For this review, take the finished solid that the model builds, in its own axes (mm). Face numbers are marked on the shaded views. Coordinates: 2 decimals unless noted, no trailing zeros. Write each loop counter-clockwise with the first axis right and the second up, starting at its lowest first coordinate (ties: lowest second). Pieces come first, ordered by that corner, then holes. Notation, with made-up numbers: (58.25, -11.5) -> (73.25, -11.5) arc R26 ccw to (73.25, 26.5) -> close; hole circle Ø11 at (-34.5, -9.75). An arc over 180 degrees is marked (long way). Put each result on its own line as item: value. Start each with the question number.
Item 1: To check wall thickness, follow L1, parallel to Y at x = -19, z = 2.95; L2, parallel to Z at x = 49.5, y = 0.9; L3, parallel to X at y = -32, z = 2. State the ranges of each line that lie inside material, in increasing order.
Item 2: Consider section B-B on y = 12. Give the boundary of the cut face in (x, z), and give its area (3 significant figures).
Item 3: Consider section C-C on x = -37. Give the boundary of the cut face in (y, z).
Item 4: Consider section A-A on z = 2.75. Give the boundary of the cut face in (x, y).
Item 5: Insertion check: P1, Ø1.5, axis at x = 49, z = 4, coming from the -Y side; P2, Ø1.2, axis at y = -8, z = 3, coming from the +X side; P3, Ø1.5, axis at x = 49.5, z = 3.5, coming from the +Y side; P4, Ø4, axis at x = -1.5, y = 33.5, coming from the -Z side. Each pin has a flat end and moves straight along its axis. Give the tip position at first contact, or say it passes through.
Item 6: The part is to be moulded in two halves that separate along Y. For the marked faces 1 and 2, say which applies: +Y half, -Y half, draft (parallel to the pull), parting line (faces both ways), or undercut.
```python
from build123d import *

# Parameters (mm, degrees)
SKETCH1_W           = 88
SKETCH1_H           = 103
BOSS_EXTRUDE1_DEPTH = 5.5
SHELL1_T            = -1.25
SKETCH2_W           = 5
SKETCH2_H           = 10
BOSS_EXTRUDE2_DEPTH = 8
FILLET1_RADIUS      = 2.5
FILLET1_LENGTH      = 10
SKETCH3_R           = 1.5
CUT_EXTRUDE1_DEPTH  = 3
FILLET2_R           = 1.5


with BuildPart() as part:
    # Sketch1 → Boss-Extrude1 (new body)
    with BuildSketch(Plane.XY):
        Rectangle(SKETCH1_W, SKETCH1_H)
    extrude(amount=BOSS_EXTRUDE1_DEPTH)

    # Shell1
    shell1_openings = [part.faces().sort_by_distance(p)[0] for p in [
        (0, 0, 5.5),
    ]]
    offset(amount=SHELL1_T, openings=shell1_openings, kind=Kind.INTERSECTION)

    # Sketch2 → Boss-Extrude2 (add)
    with BuildSketch(Plane(origin=(44, 0, 0), x_dir=(0, 0, -1), z_dir=(1, 0, 0))):
        with Locations((-2.75, 5)):
            Rectangle(SKETCH2_W, SKETCH2_H)
    extrude(amount=BOSS_EXTRUDE2_DEPTH)

    # Fillet1: full round fillet: the end face becomes a half cylinder, R = half its width
    fillet1_face = Plane((52, 5, 2.75), x_dir=(0, 1, 0), z_dir=(1, 0, 0))  # on the end face: x along it, z out of the body
    fillet1_slab = fillet1_face.offset(-FILLET1_RADIUS / 2) * Box(FILLET1_LENGTH, 2 * FILLET1_RADIUS, FILLET1_RADIUS, mode=Mode.PRIVATE)  # the body's end, R deep
    fillet1_round = Plane((49.5, 5, 2.75), x_dir=(1, 0, 0), z_dir=(0, 1, 0)) * Cylinder(FILLET1_RADIUS, FILLET1_LENGTH, mode=Mode.PRIVATE)  # its axis R under the face
    add(fillet1_slab - fillet1_round, mode=Mode.SUBTRACT)

    # Sketch3 → Cut-Extrude1 (cut)
    with BuildSketch(Plane.XZ):
        with Locations((49.5, 2.75)):
            Circle(SKETCH3_R)
    extrude(amount=-CUT_EXTRUDE1_DEPTH, mode=Mode.SUBTRACT)

    # Fillet2
    # the kernel refuses this fillet: 1.5 mm, written as the material it takes off along each edge
    with BuildSketch(Plane(origin=(-42.5, -50, 1.5), x_dir=(0, 0, -1), z_dir=(-1, 0, 0))) as fillet2_piece_1_section:
        Polygon((0, 0), (FILLET2_R, 0), (FILLET2_R, FILLET2_R), (0, FILLET2_R), align=None)
    fillet2_piece_1 = extrude(amount=FILLET2_R, mode=Mode.PRIVATE)
    fillet2_piece_1 = fillet2_piece_1 - Plane(origin=(-42.5, -50, 1.5), x_dir=(0, 0.7071067811865475, 0.7071067811865475), z_dir=(-1, 0, 0)) * Sphere(FILLET2_R, mode=Mode.PRIVATE)
    add(fillet2_piece_1, mode=Mode.SUBTRACT)
    with BuildSketch(Plane(origin=(-42.5, 50, 1.5), x_dir=(-1, 0, 0), z_dir=(0, 1, 0))) as fillet2_piece_2_section:
        Polygon((0, 0), (FILLET2_R, 0), (FILLET2_R, -FILLET2_R), (0, -FILLET2_R), align=None)
    fillet2_piece_2 = extrude(amount=FILLET2_R, mode=Mode.PRIVATE)
    fillet2_piece_2 = fillet2_piece_2 - Plane(origin=(-42.5, 50, 1.5), x_dir=(0.7071067811865475, 0, 0.7071067811865475), z_dir=(0, 1, 0)) * Sphere(FILLET2_R, mode=Mode.PRIVATE)
    add(fillet2_piece_2, mode=Mode.SUBTRACT)
    with BuildSketch(Plane(origin=(42.5, -50, 1.5), x_dir=(0, 0, -1), z_dir=(1, 0, 0))) as fillet2_piece_3_section:
        Polygon((0, 0), (FILLET2_R, 0), (FILLET2_R, -FILLET2_R), (0, -FILLET2_R), align=None)
    fillet2_piece_3 = extrude(amount=FILLET2_R, mode=Mode.PRIVATE)
    fillet2_piece_3 = fillet2_piece_3 - Plane(origin=(42.5, -50, 1.5), x_dir=(0, 0.7071067811865475, 0.7071067811865475), z_dir=(1, 0, 0)) * Sphere(FILLET2_R, mode=Mode.PRIVATE)
    add(fillet2_piece_3, mode=Mode.SUBTRACT)
    with BuildSketch(Plane(origin=(42.5, 50, 1.5), x_dir=(1, 0, 0), z_dir=(0, 1, 0))) as fillet2_piece_4_section:
        Polygon((0, 0), (FILLET2_R, 0), (FILLET2_R, FILLET2_R), (0, FILLET2_R), align=None)
    fillet2_piece_4 = extrude(amount=FILLET2_R, mode=Mode.PRIVATE)
    fillet2_piece_4 = fillet2_piece_4 - Plane(origin=(42.5, 50, 1.5), x_dir=(-0.7071067811865475, 0, 0.7071067811865475), z_dir=(0, 1, 0)) * Sphere(FILLET2_R, mode=Mode.PRIVATE)
    add(fillet2_piece_4, mode=Mode.SUBTRACT)
    with BuildSketch(Plane(origin=(-44, -50, 0), x_dir=(0, 0, 1), z_dir=(0, 1, 0))) as fillet2_piece_5:
        with BuildLine():
            CenterArc((FILLET2_R, FILLET2_R), FILLET2_R, 180, 90)
            Line((0, FILLET2_R), (0, 0))
            Line((0, 0), (FILLET2_R, 0))
        make_face()
    extrude(amount=100, mode=Mode.SUBTRACT)
    with BuildSketch(Plane(origin=(42.5, -51.5, 0), x_dir=(0, 1, 0), z_dir=(-1, 0, 0))) as fillet2_piece_6:
        with BuildLine():
            CenterArc((FILLET2_R, -FILLET2_R), FILLET2_R, 90, 90)
            Line((0, -FILLET2_R), (0, 0))
            Line((0, 0), (FILLET2_R, 0))
        make_face()
    extrude(amount=85, mode=Mode.SUBTRACT)
    with BuildSketch(Plane(origin=(44, 50, 0), x_dir=(0, 0, 1), z_dir=(0, -1, 0))) as fillet2_piece_7_section:
        with BuildLine():
            CenterArc((FILLET2_R, FILLET2_R), FILLET2_R, 180, 90)
            Line((0, FILLET2_R), (0, 0))
            Line((0, 0), (FILLET2_R, 0))
        make_face()
    fillet2_piece_7 = extrude(amount=100, mode=Mode.PRIVATE)
    fillet2_piece_7 = split(fillet2_piece_7, bisect_by=Plane(origin=(43.836700162, 30, 0.25), z_dir=(0, 0, 1)), keep=Keep.TOP, mode=Mode.PRIVATE)
    fillet2_piece_7 = split(fillet2_piece_7, bisect_by=Plane(origin=(43.836700162, 10, 0.589852414), z_dir=(0, 1, 0)), keep=Keep.TOP, mode=Mode.PRIVATE)
    add(fillet2_piece_7, mode=Mode.SUBTRACT)
    with BuildSketch(Plane(origin=(44, 50, 0), x_dir=(0, 0, 1), z_dir=(0, -1, 0))) as fillet2_piece_8_section:
        with BuildLine():
            CenterArc((FILLET2_R, FILLET2_R), FILLET2_R, 180, 90)
            Line((0, FILLET2_R), (0, 0))
            Line((0, 0), (FILLET2_R, 0))
        make_face()
    fillet2_piece_8 = extrude(amount=100, mode=Mode.PRIVATE)
    fillet2_piece_8 = split(fillet2_piece_8, bisect_by=Plane(origin=(43.48515527, 30, 0.25), z_dir=(0, 0, -1)), keep=Keep.TOP, mode=Mode.PRIVATE)
    fillet2_piece_8 = split(fillet2_piece_8, bisect_by=Plane(origin=(43.48515527, 10, 0.09081038), z_dir=(0, 1, 0)), keep=Keep.TOP, mode=Mode.PRIVATE)
    add(fillet2_piece_8, mode=Mode.SUBTRACT)
    with BuildSketch(Plane(origin=(44, 50, 0), x_dir=(0, 0, 1), z_dir=(0, -1, 0))) as fillet2_piece_9_section:
        with BuildLine():
            CenterArc((FILLET2_R, FILLET2_R), FILLET2_R, 180, 90)
            Line((0, FILLET2_R), (0, 0))
            Line((0, 0), (FILLET2_R, 0))
        make_face()
    fillet2_piece_9 = extrude(amount=100, mode=Mode.PRIVATE)
    fillet2_piece_9 = split(fillet2_piece_9, bisect_by=Plane(origin=(43.48515527, 0, 0.09081038), z_dir=(0, 1, 0)), keep=Keep.TOP, mode=Mode.PRIVATE)
    fillet2_piece_9 = split(fillet2_piece_9, bisect_by=Plane(origin=(43.48515527, 5, 0.25), z_dir=(0, 0, -1)), keep=Keep.TOP, mode=Mode.PRIVATE)
    fillet2_piece_9 = split(fillet2_piece_9, bisect_by=Plane(origin=(43.48515527, 10, 0.09081038), z_dir=(0, -1, 0)), keep=Keep.TOP, mode=Mode.PRIVATE)
    add(fillet2_piece_9, mode=Mode.SUBTRACT)
    with BuildSketch(Plane(origin=(44, 50, 0), x_dir=(0, 0, 1), z_dir=(0, -1, 0))) as fillet2_piece_10_section:
        with BuildLine():
            CenterArc((FILLET2_R, FILLET2_R), FILLET2_R, 180, 90)
            Line((0, FILLET2_R), (0, 0))
            Line((0, 0), (FILLET2_R, 0))
        make_face()
    fillet2_piece_10 = extrude(amount=100, mode=Mode.PRIVATE)
    fillet2_piece_10 = split(fillet2_piece_10, bisect_by=Plane(origin=(43.836700162, 0, 0.589852414), z_dir=(0, -1, 0)), keep=Keep.TOP, mode=Mode.PRIVATE)
    fillet2_piece_10 = split(fillet2_piece_10, bisect_by=Plane(origin=(43.836700162, -25, 0.25), z_dir=(0, 0, 1)), keep=Keep.TOP, mode=Mode.PRIVATE)
    add(fillet2_piece_10, mode=Mode.SUBTRACT)
    with BuildSketch(Plane(origin=(44, 50, 0), x_dir=(0, 0, 1), z_dir=(0, -1, 0))) as fillet2_piece_11_section:
        with BuildLine():
            CenterArc((FILLET2_R, FILLET2_R), FILLET2_R, 180, 90)
            Line((0, FILLET2_R), (0, 0))
            Line((0, 0), (FILLET2_R, 0))
        make_face()
    fillet2_piece_11 = extrude(amount=100, mode=Mode.PRIVATE)
    fillet2_piece_11 = split(fillet2_piece_11, bisect_by=Plane(origin=(43.48515527, 0, 0.09081038), z_dir=(0, -1, 0)), keep=Keep.TOP, mode=Mode.PRIVATE)
    fillet2_piece_11 = split(fillet2_piece_11, bisect_by=Plane(origin=(43.48515527, -25, 0.25), z_dir=(0, 0, -1)), keep=Keep.TOP, mode=Mode.PRIVATE)
    add(fillet2_piece_11, mode=Mode.SUBTRACT)
    with BuildSketch(Plane(origin=(-42.5, 51.5, 0), x_dir=(0, 0, 1), z_dir=(1, 0, 0))) as fillet2_piece_12:
        with BuildLine():
            CenterArc((FILLET2_R, FILLET2_R), FILLET2_R, 180, 90)
            Line((0, FILLET2_R), (0, 0))
            Line((0, 0), (FILLET2_R, 0))
        make_face()
    extrude(amount=85, mode=Mode.SUBTRACT)
    with BuildSketch(Plane(origin=(44, 51.5, 1.5), x_dir=(-1, 0, 0), z_dir=(0, 0, 1)), Plane(origin=(44, -51.5, 1.5), x_dir=(0, 1, 0), z_dir=(0, 0, 1))) as fillet2_piece_13:
        with BuildLine():
            CenterArc((FILLET2_R, FILLET2_R), FILLET2_R, 180, 90)
            Line((0, FILLET2_R), (0, 0))
            Line((0, 0), (FILLET2_R, 0))
        make_face()
    extrude(amount=7.75, mode=Mode.SUBTRACT)
    with BuildSketch(Plane(origin=(-44, -51.5, 1.5), x_dir=(0, 1, 0), z_dir=(0, 0, 1)), Plane(origin=(-44, 51.5, 1.5), x_dir=(1, 0, 0), z_dir=(0, 0, 1))) as fillet2_piece_14:
        with BuildLine():
            CenterArc((FILLET2_R, -FILLET2_R), FILLET2_R, 90, 90)
            Line((0, -FILLET2_R), (0, 0))
            Line((0, 0), (FILLET2_R, 0))
        make_face()
    extrude(amount=7.75, mode=Mode.SUBTRACT)


solid = part.part
```
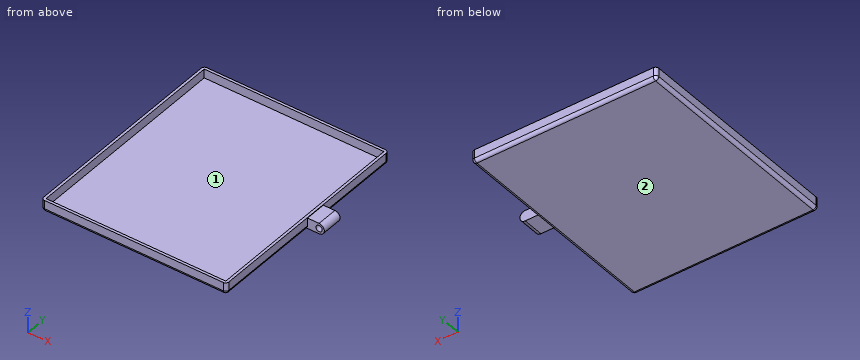
Return value:
1. L1: -51.5 to -50.25, 50.25 to 51.5
1. L2: 0.25 to 1.25, 4.25 to 5.25
1. L3: -44 to -42.75, 42.75 to 44
2. outline: (-44, 1.5) arc R1.5 ccw to (-42.5, 0) -> (42.5, 0) arc R1.5 ccw to (44, 1.5) -> (44, 5.5) -> (42.75, 5.5) -> (42.75, 1.25) -> (-42.75, 1.25) -> (-42.75, 5.5) -> (-44, 5.5) -> close
2. area: 120 mm^2
3. outline: (-51.5, 1.5) arc R1.5 ccw to (-50, 0) -> (50, 0) arc R1.5 ccw to (51.5, 1.5) -> (51.5, 5.5) -> (50.25, 5.5) -> (50.25, 1.25) -> (-50.25, 1.25) -> (-50.25, 5.5) -> (-51.5, 5.5) -> close
4. outline: (-44, -50) arc R1.5 ccw to (-42.5, -51.5) -> (42.5, -51.5) arc R1.5 ccw to (44, -50) -> (44, 0) -> (48, 0) -> (48, 3) -> (51, 3) -> (51, 0) -> (52, 0) -> (52, 10) -> (44, 10) -> (44, 50) arc R1.5 ccw to (42.5, 51.5) -> (-42.5, 51.5) arc R1.5 ccw to (-44, 50) -> close; hole (-42.75, -50.25) -> (42.75, -50.25) -> (42.75, 50.25) -> (-42.75, 50.25) -> close
5. P1: y = 0
5. P2: x = 44
5. P3: y = 10
5. P4: z = 0
6. face 1: undercut
6. face 2: draft
